Geometry check sheet. Reference: the model listing, model coordinates, mm. A direction names the side the tool comes from. Coordinates: 2 decimals unless noted, no trailing zeros. Write each loop counter-clockwise with the first axis right and the second up, starting at its lowest first coordinate (ties: lowest second). Pieces come first, ordered by that corner, then holes. Notation, with made-up numbers: M 84.5,48 L 117.5,48 A25 cw 117.5,86 Z; hole C 63,-1.5 d4. An arc over 180 degrees is marked long. Write each question's results on one line, items separated by ' | '.
```python
from build123d import *

# Parameters (mm, degrees)
SKETCH1_W                           = 50.8
SKETCH1_H                           = 25.4
BOSS_EXTRUDE1_DEPTH                 = 22.225
SKETCH2_R                           = 9.525
CUT_EXTRUDE1_DEPTH                  = 26.4
SKETCH4_W                           = 44.45
SKETCH4_H                           = 19.05
CUT_EXTRUDE3_DEPTH                  = 45.45
F_9_64_0_14063_DIAMETER_HOLE2_D     = 3.572002
F_9_64_0_14063_DIAMETER_HOLE2_DEPTH = 3.175
F_5_32_0_15625_DIAMETER_HOLE1_D     = 3.96875
F_5_32_0_15625_DIAMETER_HOLE1_DEPTH = 3.175


with BuildPart() as part:
    # Sketch1 → Boss-Extrude1 (new body, symmetric)
    with BuildSketch(Plane.XY):
        with Locations((0, 12.7)):
            Rectangle(SKETCH1_W, SKETCH1_H)
    extrude(amount=BOSS_EXTRUDE1_DEPTH, both=True)

    # Sketch2 → Cut-Extrude1 (cut, through all)
    with BuildSketch(Plane(origin=(0, 25.4, 0), x_dir=(1, 0, 0), z_dir=(0, 1, 0))):
        Circle(SKETCH2_R)
    extrude(amount=-CUT_EXTRUDE1_DEPTH, mode=Mode.SUBTRACT)

    # Sketch4 → Cut-Extrude3 (cut, through all)
    with BuildSketch(Plane(origin=(0, 0, -22.225), x_dir=(-1, 0, 0), z_dir=(0, 0, -1))):
        with Locations((0, 12.7)):
            Rectangle(SKETCH4_W, SKETCH4_H)
    extrude(amount=-CUT_EXTRUDE3_DEPTH, mode=Mode.SUBTRACT)

    # 9/64 (0.14063) Diameter Hole2
    with Locations(Plane(origin=(0, 25.4, 0), x_dir=(1, 0, 0), z_dir=(0, 1, 0))):
        with Locations((-13.470384182, 13.470384182), (13.470384182, 13.470384182), (13.470384182, -13.470384182), (-13.470384182, -13.470384182)):
            Hole(F_9_64_0_14063_DIAMETER_HOLE2_D / 2, depth=F_9_64_0_14063_DIAMETER_HOLE2_DEPTH)

    # 5/32 (0.15625) Diameter Hole1
    with Locations(Plane(origin=(0, 0, 0), x_dir=(-1, 0, 0), z_dir=(0, -1, 0))):
        with Locations((-12.727922061, 12.727922061), (12.727922061, 12.727922061), (12.727922061, -12.727922061), (-12.727922061, -12.727922061)):
            Hole(F_5_32_0_15625_DIAMETER_HOLE1_D / 2, depth=F_5_32_0_15625_DIAMETER_HOLE1_DEPTH)


solid = part.part
```
Q1. Sectioned sample at B-B on y = 8. Record the cut outline in (x, z) (3 decimals), and give its area (3 significant figures).
Geometry check:
outline: M -25.4,-22.225 L -22.225,-22.225 L -22.225,22.225 L -25.4,22.225 Z; M 22.225,-22.225 L 25.4,-22.225 L 25.4,22.225 L 22.225,22.225 Z | area: 282 mm2
Q2. Mould release check, pull along X, two halves, no side actions. Record for faces 6 (the flat face through (0, 23, 22.225)), 7 (the flat face through (25.4, 13, 0)), 8 (the cylindrical face through (-14.295, 23.79, -11.886)): pulls with the +X half, pulls with the -X half, needs draft (parallel to the pull), parting line crosses it, or undercut.
Geometry check:
face 6: needs draft | face 7: pulls with the +X half | face 8: undercut
Q3. Sectioned sample at C-C on z = 0. Record the cut outline in (x, y) (3 decimals).
Geometry check:
outline: M -25.4,0 L -9.525,0 L -9.525,3.175 L -22.225,3.175 L -22.225,22.225 L -9.525,22.225 L -9.525,25.4 L -25.4,25.4 Z; M 9.525,0 L 25.4,0 L 25.4,25.4 L 9.525,25.4 L 9.525,22.225 L 22.225,22.225 L 22.225,3.175 L 9.525,3.175 Z
Q4. Scan lines: probe 1 along Y at (x, z) = (-13, 20) (3 decimals); probe 2 along X at (y, z) = (3.25, 5) (3 decimals); probe 3 along Z at (x, y) = (0, 1) (3 decimals). Record each from-to range of solid material in increasing order.
Geometry check:
probe 1: y = 0 to 3.175, 22.225 to 25.4 | probe 2: x = -25.4 to -22.225, 22.225 to 25.4 | probe 3: z = -22.225 to -9.525, 9.525 to 22.225
Q5. Depth check by flat-ended pin: P1, Ø6, axis at x = 14, y = 7.5, coming from the -Z side; P2, Ø3, axis at x = -12.73, z = -12.73, coming from the -Y side (3 decimals); P3, Ø2, axis at x = 13.47, z = -13.47, coming from the +Y side (3 decimals). Enter the tip coordinate at first touch or a pass-through.
Geometry check:
P1: passes through | P2: stops at y = 22.225 | P3: stops at y = 3.175
Q6. Sectioned sample at D-D on x = 0. Record the cut outline in (y, z) (3 decimals), and give its area (3 significant figures).
Geometry check:
outline: M 0,-22.225 L 3.175,-22.225 L 3.175,-9.525 L 0,-9.525 Z; M 0,9.525 L 3.175,9.525 L 3.175,22.225 L 0,22.225 Z; M 22.225,-22.225 L 25.4,-22.225 L 25.4,-9.525 L 22.225,-9.525 Z; M 22.225,9.525 L 25.4,9.525 L 25.4,22.225 L 22.225,22.225 Z | area: 161 mm2
Q7. Sectioned sample at A-A on x = 20. Record the cut outline in (y, z) (3 decimals).
Geometry check:
outline: M 0,-22.225 L 3.175,-22.225 L 3.175,22.225 L 0,22.225 Z; M 22.225,-22.225 L 25.4,-22.225 L 25.4,22.225 L 22.225,22.225 Z
Q8. Access from +Z, -Z, +X, -X, +Y, -Y to the whole of each face (thin tool, end or side, straight path). Record for faces 1 (the flat face through (-22.225, 13, 0)), 2 (the cylindrical face through (11.153, 1.61, 13.935)), 3 (the cylindrical face through (-14.295, 23.79, 15.055)), 4 (the cylindrical face through (-7.559, 23.835, 5.796)), 5 (the flat face through (0, 23, -22.225)).
Geometry check:
face 1: +Z, -Z | face 2: -Y | face 3: +Y | face 4: +Y, -Y | face 5: -Z, +X, -X, +Y, -Y
